Read the model definition and answer for the solid it produces. Units are mm, in the model's axes. A direction names the side the tool comes from. Coordinates: 2 decimals unless noted, no trailing zeros. Write each loop counter-clockwise with the first axis right and the second up, starting at its lowest first coordinate (ties: lowest second). Pieces come first, ordered by that corner, then holes. Notation, with made-up numbers: (-30.5, 40.5) -> (2.5, 40.5) arc R20 cw to (2.5, 47.5) -> close; hole circle Ø6 at (-11, -7). An arc over 180 degrees is marked (long way). Write item = value, one per line. Start each with the question number.
1) Find the intervals of material crossed by line 1 along Y through (x, z) = (0, 12.3); line 2 along Y through (x, z) = (0, 2.75); line 3 along X through (y, z) = (-4.5, 5.25), in increasing order. Write a range as from..to.
2) For a pull along X with two mould halves and no side action, classify faces 3 (the face through (-1.333, -6.004, 3.574)), 4 (the face through (9.3, -9.3, 14.25)), 5 (the face through (12.932, -5.362, 9.32)), 6 (the face through (3.95, -6.04, 8.52)) as released by +X, released by -X, zero draft, split by the parting line, or undercut.
3) Section A-A (z = 8.25) is taken. Determine the outline of the cut face in (x, y), plus the area to 3 significant figures.
4) Flat-ended cylindrical pins translate along their axes: pin 1 Ø12 at (x, y) = (0, 12) entering from -Z; pin 2 Ø1 at (x, y) = (8.5, -7) entering from -Z; pin 3 Ø6 at (y, z) = (2, 11) entering from +X; pin 4 Ø1.5 at (x, z) = (3.5, 6.5) entering from -Y. Find the tip coordinate at first contact, or state that the pin passes through.
5) Section B-B (z = 12) is taken. Determine the outline of the cut face in (x, y).
6) A tool of negligible diameter and unlimited length cuts with its end or side. For faces 1 (the face through (-13.887, -10.648, 3.141)), 2 (the face through (3, -6, 7.25)), from which of +Z, -Z, +X, -X, +Y, -Y can it reach the whole face along a straight path? Write none if from no direction.
from build123d import *

# Parameters (mm, degrees)
CUT_EXTRUDE2_DEPTH = 7
SKETCH2_R          = 13
CUT_EXTRUDE1_DEPTH = 4.5


with BuildPart() as part:
    # Sketch1 → Revolve1 (revolve)
    with BuildSketch(Plane(origin=(0, 0, 0), x_dir=(1, 0, 0), z_dir=(0, 1, 0))):
        with BuildLine():
            Line((6.15, -14.25), (6.15, 0))
            Line((6.15, 0), (8, 0))
            ThreePointArc((8, 0), (12.85412196, -0.505420691), (17.5, -2))
            Line((17.5, -2), (17.5, -4.25))
            Line((17.5, -4.25), (14, -4.25))
            Line((14, -4.25), (14, -14.25))
            Line((14, -14.25), (6.15, -14.25))
        make_face()
    revolve(axis=Axis((0, 0, 0), (0, 0, 1)))

    # Sketch3 → Cut-Extrude2 (cut)
    with BuildSketch(Plane.XY.offset(14.25)):
        Polygon((0.608498328, -8.31690962), (7.38466563, -3.702054257), (6.776167302, 4.473706449), (-0.608498328, 8.034611791), (-7.38466563, 3.419756428), (-6.776167302, -4.756004278), align=None)
    extrude(amount=-CUT_EXTRUDE2_DEPTH, mode=Mode.SUBTRACT)

    # Sketch2 → Cut-Extrude1 (cut)
    with BuildSketch(Plane.XY.offset(14.25)):
        Circle(SKETCH2_R)
    extrude(amount=-CUT_EXTRUDE1_DEPTH, mode=Mode.SUBTRACT)


solid = part.part
Answer key:
q1.line_1 = -14..-13, 13..14
q1.line_2 = -17.5..-6.15, 6.15..17.5
q1.line_3 = -13.26..-4.19, 4.19..13.26
q2.face_3 = undercut
q2.face_4 = zero draft
q2.face_5 = split by the parting line
q2.face_6 = undercut
q3.outline = circle Ø28 at (0, 0); hole (-7.38, 3.42) -> (-6.78, -4.76) -> (0.61, -8.32) -> (7.38, -3.7) -> (6.78, 4.47) -> (-0.61, 8.03) -> close
q3.area = 441 mm^2
q4.pin_1 = 0
q4.pin_2 = 0.13
q4.pin_3 = 14
q4.pin_4 = -13.73
q5.outline = circle Ø28 at (0, 0); hole circle Ø26 at (0, 0)
q6.face_1 = +Z, -Z
q6.face_2 = +Z
